Answer from the drawing. Dimensions are ordinates in mm from the lowest x, y and z of the part. A direction names the side the tool comes from. Round coordinates to 2 decimals unless told otherwise and drop trailing zeros. Loops run counter-clockwise (first coordinate to the right, second up) from the corner with the lowest first, then second, coordinate; pieces in that order, holes last. Notation, with made-up numbers: (-10, 35) - (38, 35) arc R27 cw to (38, 51) - close; hole circle Ø9 at (77, -30). An arc over 180 degrees is marked (long way). Answer as CSV lines item,"result". Start each with the question number.
Q1. Each of these flat-tipped pins is pushed along its axis until it touches: pin 1 Ø8 at (x, z) = (64.5, 19) entering from +Y; pin 2 Ø6 at (y, z) = (3.5, 19.5) entering from +X; pin 3 Ø3 at (y, z) = (18.5, 15) entering from -X. Where does it stop, or does it pass through?
Q2. Section A-A on x = 44 is taken. Write down the section's boundary in (y, z), then the cut area to 3 significant figures.
Q3. Straight lines are drawn through the part: L1, parallel to Z at x = 44, y = 23; L2, parallel to Y at x = 72, z = 13.5; L3, parallel to X at y = 28.75, z = 24.25 (1 decimal). For each, find the intervals that lie inside material, in ascending order. Write a range as [from, to].
Q4. For the marked faces 1, 2 and 3, determine the directions among +Z, -Z, +X, -X, +Y, -Y from which every point of the face is accessible in a straight line to the end or side of a thin tool.
Q5. Section B-B on z = 6 is taken. Write down the section's boundary in (x, y), then the cut area to 3 significant figures.
Q6. Section C-C on y = 2.5 is taken. Write down the section's boundary in (x, z), then the cut area to 3 significant figures.
Q7. Section D-D on x = 12 is taken. Write down the section's boundary in (y, z), then the cut area to 3 significant figures.
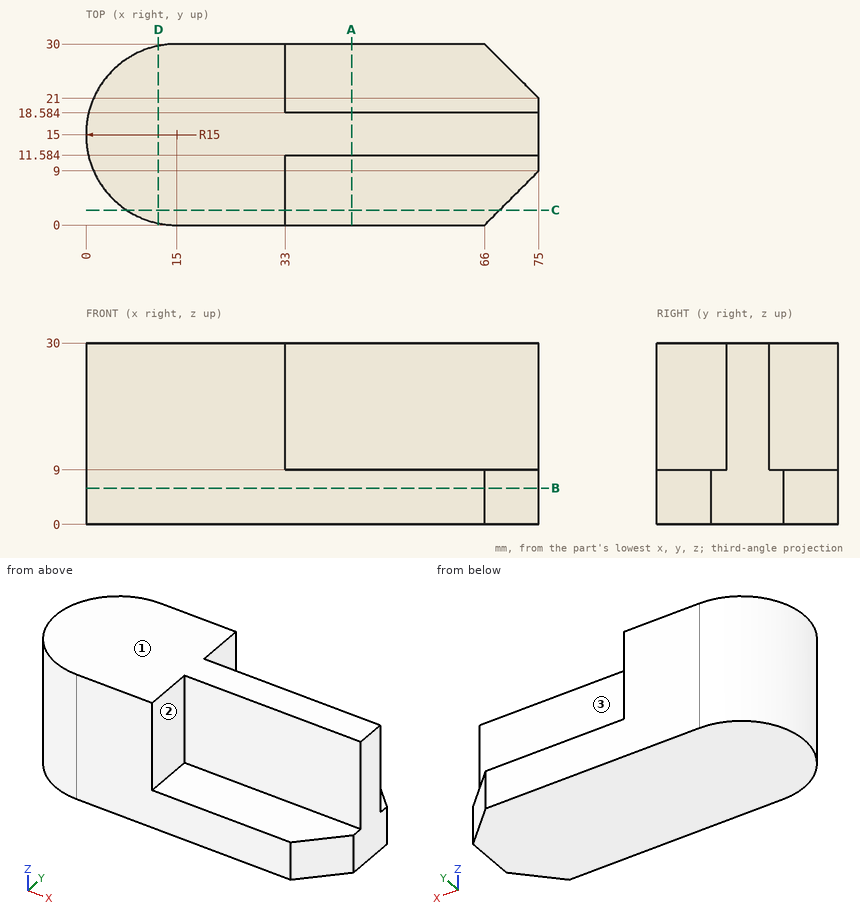
Findings:
1,pin 1,"stops at y = 18.58"
1,pin 2,"stops at x = 33"
1,pin 3,"stops at x = 0.13"
2,outline,"(0, 0) - (30, 0) - (30, 9) - (18.58, 9) - (18.58, 30) - (11.58, 30) - (11.58, 9) - (0, 9) - close"
2,area,"417 mm^2"
3,L1,"z = [0, 9]"
3,L2,"y = [11.58, 18.58]"
3,L3,"x = [9, 33]"
4,face 1,"+Z, +X, -X, +Y, -Y"
4,face 2,"+Z, +X, -Y"
4,face 3,"+Z, +X, +Y"
5,outline,"(15, 0) - (66, 0) - (75, 9) - (75, 21) - (66, 30) - (15, 30) arc R15 ccw to start"
5,area,"2,070 mm^2"
6,outline,"(6.71, 0) - (68.5, 0) - (68.5, 9) - (33, 9) - (33, 30) - (6.71, 30) - close"
6,area,"1,110 mm^2"
7,outline,"(0.3, 0) - (29.7, 0) - (29.7, 30) - (0.3, 30) - close"
7,area,"882 mm^2"
